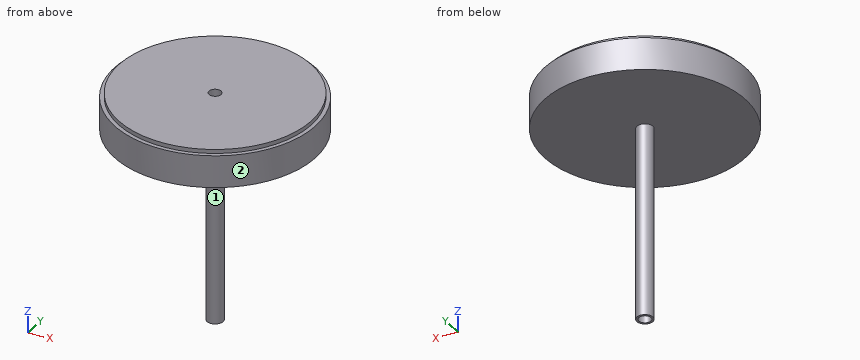
```python
from build123d import *

# Parameters (mm, degrees)
F0_R     = 152.4
F1_DEPTH = 6.35
F2_R     = 158.75
F3_DEPTH = 50.8
F4_R     = 6.35
F5_DEPTH = 57.151
F6_R     = 12.7
F7_DEPTH = 304.8
F8_R     = 9.525
F9_DEPTH = 361.951


with BuildPart() as f1:
    # F0 (on Top) → F1 (new body)
    with BuildSketch(Plane.XY):
        Circle(F0_R)
    extrude(amount=-F1_DEPTH)

    # F2 (on face) → F3 (join)
    with BuildSketch(Plane(origin=(0, 0, -6.35), x_dir=(1, 0, 0), z_dir=(0, 0, -1))):
        Circle(F2_R)
    extrude(amount=F3_DEPTH)

    # F4 (on face) → F5 (cut, through all)
    with BuildSketch(Plane.XY):
        Circle(F4_R)
    extrude(amount=-F5_DEPTH, mode=Mode.SUBTRACT)

    # F6 (on face) → F7 (join)
    with BuildSketch(Plane(origin=(0, 0, -57.15), x_dir=(1, 0, 0), z_dir=(0, 0, -1))):
        Circle(F6_R)
    extrude(amount=F7_DEPTH)

    # F8 (on face) → F9 (cut, through all)
    with BuildSketch(Plane(origin=(0, 0, -361.95), x_dir=(1, 0, 0), z_dir=(0, 0, -1))):
        Circle(F8_R)
    extrude(amount=-F9_DEPTH, mode=Mode.SUBTRACT)


solid = f1.part
```
CAD build for the part. Positions are in the model's coordinates, mm. Face numbers are marked on the shaded views. A direction names the side the tool comes from. Give positions to 0.01 mm unless a question says otherwise; leave off trailing zeros. Write each loop counter-clockwise with the first axis right and the second up, starting at its lowest first coordinate (ties: lowest second). Pieces come first, ordered by that corner, then holes. Notation, with made-up numbers: M 74,40 L 91,40 A25 ccw 91,66 Z; hole C 13,75 d11. An arc over 180 degrees is marked long. Return JSON: item names as keys, results as strings. Group by question number.
(1) Drill centre lines: L1, parallel to Y at x = 0, z = -242 (3 decimals); L2, parallel to Z at x = 73, y = 111. Where is each one in solid material? Low to high. Write a range as [from, to].
(2) 3-axis set-ups, long thin cutter, end or side, ignore diameter. For the marked faces 1 and 2: which of +Z, -Z, +X, -X, +Y, -Y reach the whole face in a straight line?
(3) Flat gauge pins, fed straight in: pin 1 Ø11.5 at (x, y) = (0, 0) entering from -Z; pin 2 Ø2 at (x, y) = (-76, -34.5) entering from -Z; pin 3 Ø6 at (x, z) = (-10.5, -253) entering from -Y; pin 4 Ø5 at (y, z) = (-6, -229.5) entering from +X. Where does each tip first touch, or does it go through?
(4) Band-saw the part on A-A (y = 0). Give the cut face in (x, z) (3 decimals), and give its area (3 significant figures).
(5) Band-saw the part on C-C (z = -317). Give the cut face in (x, y) (3 decimals), and give its area (3 significant figures).
(6) Band-saw the part on D-D (x = 99). Give the cut face in (y, z), and give its area (3 significant figures).
Entries:
{
 "1": {"L1": "y = [-12.7, -9.525], [9.525, 12.7]", "L2": "z = [-57.15, 0]"},
 "2": {"face 1": "-Z", "face 2": "+Z, -Z"},
 "3": {"pin 1": "passes through", "pin 2": "stops at z = -57.15", "pin 3": "stops at y = -10.25", "pin 4": "stops at x = 12.21"},
 "4": {"outline": "M -158.75,-57.15 L -12.7,-57.15 L -12.7,-361.95 L -9.525,-361.95 L -9.525,0 L -152.4,0 L -152.4,-6.35 L -158.75,-6.35 Z; M 9.525,-361.95 L 12.7,-361.95 L 12.7,-57.15 L 158.75,-57.15 L 158.75,-6.35 L 152.4,-6.35 L 152.4,0 L 9.525,0 Z", "area": "18,900 mm^2"},
 "5": {"outline": "C 0,0 d25.4; hole C 0,0 d19.05", "area": "222 mm^2"},
 "6": {"outline": "M -124.1,-57.15 L 124.1,-57.15 L 124.1,-6.35 L 115.87,-6.35 L 115.87,0 L -115.87,0 L -115.87,-6.35 L -124.1,-6.35 Z", "area": "14,100 mm^2"}
}
